from build123d import *

# Parameters (mm, degrees)
TAGLIO_ESTRUSIONE1_DEPTH    = 18.035037423
RIPETIZIONECIRCOLARE1_COUNT = 4


with BuildPart() as part:
    # Schizzo1 → Rivoluzione1 (revolve)
    with BuildSketch(Plane.XY, mode=Mode.PRIVATE) as rivoluzione1_sk:
        with BuildLine():
            Line((0.2, 0.851836252), (6.2, 0.851836252))
            Line((6.2, 0.851836252), (6.2, -0.851836252))
            Line((6.2, -0.851836252), (0.2, -0.851836252))
            ThreePointArc((0.2, -0.851836252), (0.875, 0), (0.2, 0.851836252))
        make_face()
    revolve(rivoluzione1_sk.sketch.rotate(Axis((7.7, 1.619035734, 0), (0, -1, 0)), 270), axis=Axis((7.7, 1.619035734, 0), (0, -1, 0)))

    # Schizzo2 → Taglio-Estrusione1 (cut, through all)
    with BuildSketch(Plane.XZ.offset(0.851836252)):
        with BuildLine():
            Line((4.335758437, 2.163764938), (3.074167851, 2.97517679))
            ThreePointArc((3.074167851, 2.97517679), (2.287737491, 0.978475617), (2.325275036, -1.167189598))
            Line((2.325275036, -1.167189598), (3.791109117, -0.848865162))
            ThreePointArc((3.791109117, -0.848865162), (3.763809084, 0.711618631), (4.335758437, 2.163764938))
        make_face()
    taglio_estrusione1 = extrude(amount=-TAGLIO_ESTRUSIONE1_DEPTH, mode=Mode.SUBTRACT)

    # RipetizioneCircolare1: Taglio-Estrusione1 ×4 about axis
    ripetizionecircolare1_axis = Axis((7.7, -0.851836252, 0), (0, 1, 0))
    for i in range(1, RIPETIZIONECIRCOLARE1_COUNT):
        add(taglio_estrusione1.rotate(ripetizionecircolare1_axis, i * 360 / RIPETIZIONECIRCOLARE1_COUNT), mode=Mode.SUBTRACT)


solid = part.part
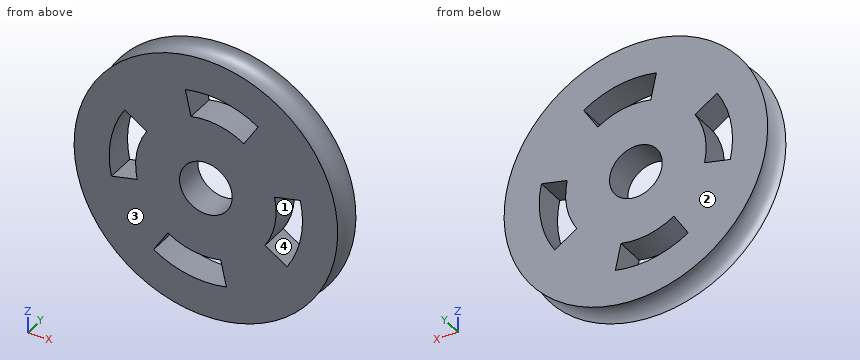
Design review of the part built by this model. Coordinates are the model's own, in mm. Face numbers are marked on the shaded views. A direction names the side the tool comes from. Round coordinates to 2 decimals unless told otherwise and drop trailing zeros. Loops run counter-clockwise (first coordinate to the right, second up) from the corner with the lowest first, then second, coordinate; pieces in that order, holes last. Notation, with made-up numbers: (67.5, -36) -> (113.5, -36) arc R15 ccw to (113.5, -8) -> close; hole circle Ø7 at (-10.5, -27.75). An arc over 180 degrees is marked (long way). Use one line per item in the form item = value. Start each with the question number.
Q1. Wall thickness on line 1 along X through (y, z) = (0.1, -0.5); line 2 along Z through (x, y) = (7.5, 0.4) (3 decimals); line 3 along Z through (x, y) = (3, -0.6): over which ranges is each line inside the solid? List them lowest first. Write a range as [from, to].
Q2. Draft analysis for pull direction Z (two halves, no side actions). For the marked faces 1 and 2, state which applies: +Z half, -Z half, draft (parallel to the pull), parting line (faces both ways), or undercut.
Q3. Machinability: for the marked faces 3 and 4, which of the approach directions +Z, -Z, +X, -X, +Y, -Y give a long, thin tool a straight path to every point of the face, cutting with its end or side? Answer none if there is none.
Q4. We need section B-B on x = 7.7. Give the boundary of the cut face in (y, z) (3 decimals).
Q5. We need section A-A on z = 0. Give the boundary of the cut face in (x, y) (3 decimals), then the cut area to 3 significant figures.
Q6. We need section C-C on y = 0.1. Give the boundary of the cut face in (x, z).
Calculated:
q1.line_1 = [0.89, 2.22], [3.73, 6.29], [9.11, 11.67], [13.18, 14.51]
q1.line_2 = [-6.919, -5.496], [-3.995, -1.487], [1.487, 3.995], [5.496, 6.919]
q1.line_3 = [-5.27, -1.02], [2.86, 5.27]
q2.face_1 = undercut
q2.face_2 = draft
q3.face_3 = +Z, -Z, +X, -X, -Y
q3.face_4 = +Y, -Y
q4.outline = (-0.852, -7.5) arc R0.875 cw to (0.852, -7.5) -> (0.852, -5.5) -> (-0.852, -5.5) -> close; (-0.852, -4) -> (0.852, -4) -> (0.852, -1.5) -> (-0.852, -1.5) -> close; (-0.852, 1.5) -> (0.852, 1.5) -> (0.852, 4) -> (-0.852, 4) -> close; (-0.852, 5.5) -> (0.852, 5.5) -> (0.852, 7.5) arc R0.875 cw to (-0.852, 7.5) -> close
q5.outline = (0.2, -0.852) -> (2.2, -0.852) -> (2.2, 0.852) -> (0.2, 0.852) arc R0.875 cw to start; (3.7, -0.852) -> (6.2, -0.852) -> (6.2, 0.852) -> (3.7, 0.852) -> close; (9.2, -0.852) -> (11.7, -0.852) -> (11.7, 0.852) -> (9.2, 0.852) -> close; (13.2, -0.852) -> (15.2, -0.852) arc R0.875 cw to (15.2, 0.852) -> (13.2, 0.852) -> close
q5.area = 13.6 mm²
q6.outline = circle Ø13.66 at (7.7, 0); hole (2.33, -1.17) -> (3.79, -0.85) arc R4 cw to (4.34, 2.16) -> (3.07, 2.98) arc R5.5 ccw to start; hole (4.72, -4.63) arc R5.5 ccw to (8.87, -5.37) -> (8.55, -3.91) arc R4 cw to (5.54, -3.36) -> close; hole circle Ø3 at (7.7, 0); hole (6.53, 5.37) -> (6.85, 3.91) arc R4 cw to (9.86, 3.36) -> (10.68, 4.63) arc R5.5 ccw to start; hole (11.06, -2.16) -> (12.33, -2.98) arc R5.5 ccw to (13.07, 1.17) -> (11.61, 0.85) arc R4 cw to start
